The drawing under review shows one solid part. Ordinate dimensions are in mm from its lowest x, y, z. A direction names the side the tool comes from. Coordinates: 2 decimals unless noted, no trailing zeros. Order: outer loops, then holes, each group sorted by start corner. A loop starts at its lowest first (then second) coordinate and runs counter-clockwise, first axis right, second up. Notation, with made-up numbers: (-2.75, 4) -> (42.25, 4) arc R8 ccw to (42.25, 14) -> close; hole circle Ø3 at (-11, 24.5). An arc over 180 degrees is marked (long way). Use a Markdown table: item, result. Add a question column.
Q1. The part is to be moulded in two halves that separate along X. For the marked faces 3, 4 and 5, say which applies: pulls with the +X half, pulls with the -X half, needs draft (parallel to the pull), parting line crosses it, or undercut.
Q2. Machinability: for the marked faces 1 and 2, which of the approach directions +Z, -Z, +X, -X, +Y, -Y give a long, thin tool a straight path to every point of the face, cutting with its end or side? Answer none if there is none.
Q3. Add section B-B (y = 43). State the section outline as (x, z) points.
Q4. Wall thickness on probe 1 along X at (y, z) = (43, 3); probe 2 along X at (y, z) = (13, 3); probe 3 along Z at (x, y) = (11.25, 38): over which ranges is each line inside the solid? List them lowest first.
Q5. Add section A-A (y = 13). State the section outline as (x, z) points.
Q6. Add section C-C (x = 1.25). State the section outline as (y, z) points.
Q7. Add section D-D (y = 29). State the section outline as (x, z) points, then the cut area to 3 significant figures.
Q8. Insertion check: pin 1 (6 mm diameter, centred on x = 3.5, y = 15.5, fed in from +Z); pin 2 (2 mm diameter, centred on x = 14, z = 26.5, fed in from +Y); pin 3 (3 mm diameter, centred on x = 11.6, y = 43, fed in from +Z). Each pin has a flat end and moves straight along its axis. Give the tip position at first contact, or say it passes through.
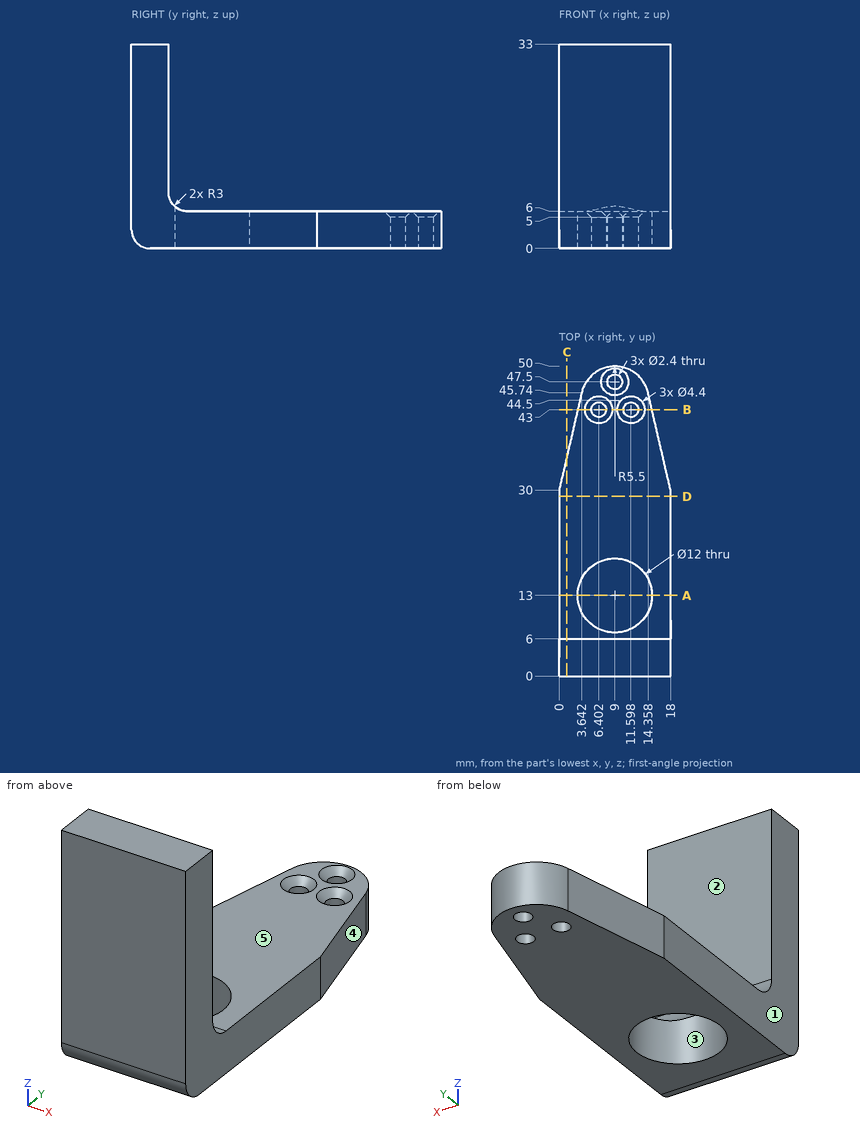
Established:
| question | item | result |
|---|---|---|
| 1 | face 3 | undercut |
| 1 | face 4 | pulls with the +X half |
| 1 | face 5 | needs draft |
| 2 | face 1 | +Z, -Z, -X, +Y, -Y |
| 2 | face 2 | +Z, +X, -X, +Y |
| 3 | outline | (3.01, 0) -> (5.2, 0) -> (5.2, 5) -> (4.2, 6) -> (3.01, 6) -> close; (7.6, 0) -> (10.4, 0) -> (10.4, 5) -> (9.4, 6) -> (8.6, 6) -> (7.6, 5) -> close; (12.8, 0) -> (14.99, 0) -> (14.99, 6) -> (13.8, 6) -> (12.8, 5) -> close |
| 4 | probe 1 | 3.01 to 5.2, 7.6 to 10.4, 12.8 to 14.99 |
| 4 | probe 2 | 0 to 3, 15 to 18 |
| 4 | probe 3 | 0 to 6 |
| 5 | outline | (0, 0) -> (3, 0) -> (3, 6) -> (0, 6) -> close; (15, 0) -> (18, 0) -> (18, 6) -> (15, 6) -> close |
| 6 | outline | (0, 3) arc R3 ccw to (3, 0) -> (35.4, 0) -> (35.4, 6) -> (9, 6) arc R3 cw to (6, 9) -> (6, 33) -> (0, 33) -> close |
| 7 | outline | (0, 0) -> (18, 0) -> (18, 6) -> (0, 6) -> close |
| 7 | area | 108 mm^2 |
| 8 | pin 1 | z = 6 |
| 8 | pin 2 | y = 6 |
| 8 | pin 3 | z = 5.3 |
